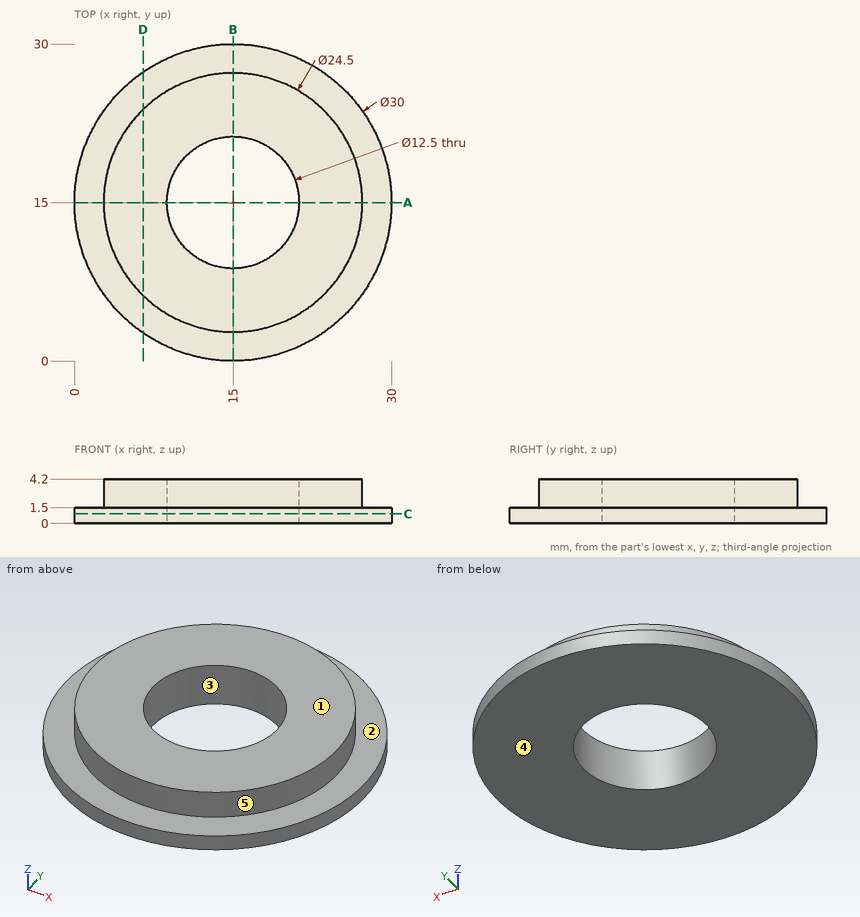
Study the drawing (mm; zero at the part's minimum x, y, z) and answer. A direction names the side the tool comes from. Round coordinates to 2 decimals unless told otherwise and drop trailing zeros. Write each loop counter-clockwise with the first axis right and the second up, starting at its lowest first coordinate (ties: lowest second). Pieces come first, ordered by that corner, then holes. Notation, with made-up numbers: (-21.75, -10) - (17.25, -10) arc R22 cw to (17.25, 29) - close; hole circle Ø7 at (86.25, 2.5). An arc over 180 degrees is marked (long way). Use CSV: the item, a comma, the result in double quotes.
Q1. Find section D-D, the plane x = 6.5. Write down the section's boundary in (y, z), then the cut area to 3 significant figures.
Values:
outline,"(2.64, 0) - (27.36, 0) - (27.36, 1.5) - (23.82, 1.5) - (23.82, 4.2) - (6.18, 4.2) - (6.18, 1.5) - (2.64, 1.5) - close"
area,"84.7 mm²"
Q2. Straight lines are drawn through the part: line 1 along X through (y, z) = (15, 0.95); line 2 along X through (y, z) = (15.25, 3.35) (3 decimals); line 3 along Y through (x, z) = (15, 3.25). For each, find the intervals that lie inside material, in ascending order.
Values:
line 1,"x = 0 to 8.75, 21.25 to 30"
line 2,"x = 2.753 to 8.755, 21.245 to 27.247"
line 3,"y = 2.75 to 8.75, 21.25 to 27.25"
Q3. Find section A-A, the plane y = 15. Write down the section's boundary in (x, z), then the cut area to 4 significant figures.
Values:
outline,"(0, 0) - (8.75, 0) - (8.75, 4.2) - (2.75, 4.2) - (2.75, 1.5) - (0, 1.5) - close; (21.25, 0) - (30, 0) - (30, 1.5) - (27.25, 1.5) - (27.25, 4.2) - (21.25, 4.2) - close"
area,"58.65 mm²"
Q4. Determine the mould class of the marked faces 3, 4 and 5 for opening direction X: +X half, -X half, draft (parallel to the pull), parting line (faces both ways), or undercut.
Values:
face 3,"undercut"
face 4,"draft"
face 5,"parting line"
Q5. A tool of negligible diameter and unlimited length cuts with its end or side. For the marked faces 1 and 2, from which of +Z, -Z, +X, -X, +Y, -Y can it reach the whole face along a straight path? Write none if from no direction.
Values:
face 1,"+Z, +X, -X, +Y, -Y"
face 2,"+Z"
Q6. Find section C-C, the plane z = 0.9. Write down the section's boundary in (x, y).
Values:
outline,"circle Ø30 at (15, 15); hole circle Ø12.5 at (15, 15)"
Q7. Each of these flat-tipped pins is pushed along its axis until it touches: pin 1 Ø2 at (x, z) = (10, 0.5) entering from -Y; pin 2 Ø14.5 at (x, y) = (15, 15) entering from -Z. Where does it stop, or does it pass through?
Values:
pin 1,"stops at y = 0.54"
pin 2,"stops at z = 0"
